from build123d import *

# Parameters (mm, degrees)
F0_W     = 20
F0_H     = 20
F1_DEPTH = 8
F2_T     = -1
F4_DEPTH = 2


with BuildPart() as f1:
    # F0 (on Top) → F1 (new body)
    with BuildSketch(Plane.XY):
        with Locations((10, 10)):
            Rectangle(F0_W, F0_H)
    extrude(amount=F1_DEPTH)

    # F2
    f2_openings = [f1.faces().sort_by_distance(p)[0] for p in [
        (20, 10, 4),
    ]]
    offset(amount=F2_T, openings=f2_openings)

    # F3 (on face) → F4 (cut)
    with BuildSketch(Plane(origin=(0, 0, 0), x_dir=(0, -1, 0), z_dir=(-1, 0, 0))):
        Polygon((-19, 7), (-19, 4.001057), (-19, 1), (-1, 1), (-1, 7), align=None)
    extrude(amount=-F4_DEPTH, mode=Mode.SUBTRACT)


solid = f1.part
Read the model definition and answer for the solid it produces. Units are mm, in the model's axes. A direction names the side the tool comes from. Round coordinates to 2 decimals unless told otherwise and drop trailing zeros. Write each loop counter-clockwise with the first axis right and the second up, starting at its lowest first coordinate (ties: lowest second). Pieces come first, ordered by that corner, then holes.
Q1. Straight lines are drawn through the part: line 1 (Z direction, x = 13, y = 10); line 2 (Y direction, x = 11, z = 5.5). For each, find the intervals that lie inside material, in ascending order.
Values:
line 1: z = 0 to 1, 7 to 8
line 2: y = 0 to 1, 19 to 20
Q2. Find section A-A on y = 2. Determine the outline of the cut face in (x, z), and give its area (3 significant figures).
Values:
outline: (0, 0) - (20, 0) - (20, 1) - (0, 1) - close; (0, 7) - (20, 7) - (20, 8) - (0, 8) - close
area: 40.0 mm2
Q3. Find section B-B on x = 4.25. Determine the outline of the cut face in (y, z), and give its area (3 significant figures).
Values:
outline: (0, 0) - (20, 0) - (20, 8) - (0, 8) - close; hole (1, 1) - (19, 1) - (19, 7) - (1, 7) - close
area: 52.0 mm2
Q4. Find section C-C on z = 3.25. Determine the outline of the cut face in (x, y).
Values:
outline: (0, 0) - (20, 0) - (20, 1) - (0, 1) - close; (0, 19) - (20, 19) - (20, 20) - (0, 20) - close
Q5. A tool of negligible diameter and unlimited length cuts with its end or side. For faces 1 (the face through (10, 10, 7)), 2 (the face through (10, 20, 4)), from which of +Z, -Z, +X, -X, +Y, -Y can it reach the whole face along a straight path? Write none if from no direction.
Values:
face 1: +X, -X
face 2: +Z, -Z, +X, -X, +Y
Q6. Flat-ended cylindrical pins translate along their axes: P1, Ø2, axis at y = 6.5, z = 4.5, coming from the -X side (1 decimal); P2, Ø1.8, axis at x = 11.5, z = 4.5, coming from the -Y side. Find the tip coordinate at first contact, or state that the pin passes through.
Values:
P1: passes through
P2: stops at y = 0
